For this review, take the finished solid that the model builds, in its own axes (mm). Face numbers are marked on the shaded views. A direction names the side the tool comes from. Round coordinates to 2 decimals unless told otherwise and drop trailing zeros. Order: outer loops, then holes, each group sorted by start corner. A loop starts at its lowest first (then second) coordinate and runs counter-clockwise, first axis right, second up. Notation, with made-up numbers: (-8, 76) -> (21, 76) arc R19 ccw to (21, 109) -> close; hole circle Ø7 at (6, 68). An arc over 180 degrees is marked (long way). Put each result on its own line as item: value. Start each with the question number.
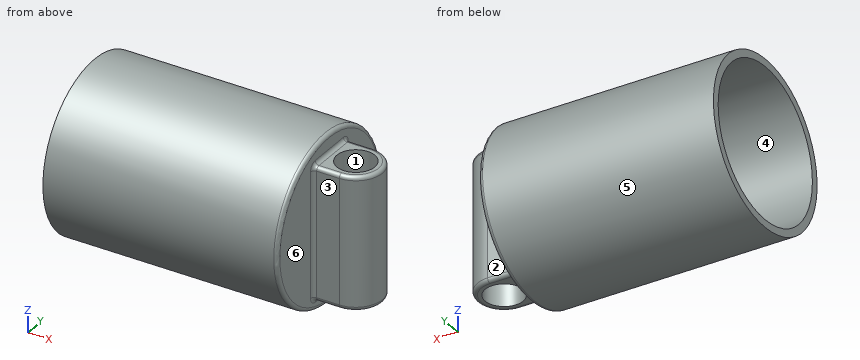
```python
from build123d import *

# Parameters (mm, degrees)
SKETCH3_R           = 5
BOSS_EXTRUDE2_DEPTH = 35
FILLET2_R           = 1
FILLET3_R           = 1


with BuildPart() as part:
    # Sketch1 → Revolve1 (revolve)
    with BuildSketch(Plane.XY, mode=Mode.PRIVATE) as revolve1_sk:
        Polygon((2, 22), (2, 0), (0, 0), (0, 20), (-60, 20), (-60, 22), align=None)
    revolve(revolve1_sk.sketch.rotate(Axis((-25.911369332, 0, 0), (1, 0, 0)), 90), axis=Axis((-25.911369332, 0, 0), (1, 0, 0)))

    # Sketch3 → Boss-Extrude2 (add)
    with BuildSketch(Plane.XY.offset(17)):
        with BuildLine():
            Line((9, 7), (2, 7))
            Line((2, 7), (2, -7))
            Line((2, -7), (9, -7))
            ThreePointArc((9, -7), (16, 0), (9, 7))
        make_face()
        with Locations((9, 0)):
            Circle(SKETCH3_R, mode=Mode.SUBTRACT)
    extrude(amount=-BOSS_EXTRUDE2_DEPTH)

    # Fillet2
    fillet2_edges = [part.edges().sort_by_distance(p)[0] for p in [
        (2, 0, -22),
    ]]
    fillet(fillet2_edges, radius=FILLET2_R)

    # Fillet3
    fillet3_edges = [part.edges().sort_by_distance(p)[0] for p in [
        (16, 0, -18),
        (5.5, -7, -18),
        (2, 0, -18),
        (2, -7, -0.5),
        (5.5, 7, -18),
        (2, 7, -0.5),
        (16, 0, 17),
        (5.5, 7, 17),
        (2, 0, 17),
        (5.5, -7, 17),
    ]]
    fillet(fillet3_edges, radius=FILLET3_R)


solid = part.part
```
Item 1: Consider section C-C, the plane x = 7.5. Write out the cut boundary in (y, z), plus the area to 3 significant figures.
Item 2: Consider section D-D, the plane x = -44. Write out the cut boundary in (y, z).
Item 3: Tool access review of the marked faces 1, 2 and 3: name each direction out of +Z, -Z, +X, -X, +Y, -Y from which nothing blocks a thin tool from reaching the whole face with its end or side.
Item 4: Consider section B-B, the plane z = 0. Write out the cut boundary in (x, y), plus the area to 3 significant figures.
Item 5: For L1, parallel to Y at x = -44.5, z = -0.5; L2, parallel to Y at x = 9, z = 7; L3, parallel to Z at x = -33, y = -18, list the stretches that pass through material, from the lowest coordinate up.
Item 6: Mouldability with a two-part tool opening along Y and no side actions: class the marked faces 4, 5 and 6 as +Y half, -Y half, draft (parallel to the pull), parting line (faces both ways), or undercut.
Item 7: Consider section A-A, the plane y = 0. Write out the cut boundary in (x, z).
Item 8: Insertion check: pin 1 Ø5 at (x, y) = (-42, 3) entering from -Z; pin 2 Ø1 at (x, y) = (-50, -13) entering from -Z; pin 3 Ø21 at (y, z) = (-9, -10.5) entering from +X; pin 4 Ø11.5 at (x, y) = (9, 0) entering from +Z. Each pin has a flat end and moves straight along its axis. Give the tip position at first contact, or say it passes through.
Evaluation:
1. outline: (-7, -17) arc R1 ccw to (-6, -18) -> (-4.77, -18) -> (-4.77, 17) -> (-6, 17) arc R1 ccw to (-7, 16) -> close; (4.77, -18) -> (6, -18) arc R1 ccw to (7, -17) -> (7, 16) arc R1 ccw to (6, 17) -> (4.77, 17) -> close
1. area: 155 mm^2
2. outline: circle Ø44 at (0, 0); hole circle Ø40 at (0, 0)
3. face 1: +Z, -Z
3. face 2: +Z, -Z, +X, +Y
3. face 3: +Z, -Z, +X, -Y
4. outline: (-60, -22) -> (1, -22) arc R1 ccw to (2, -21) -> (2, -8) arc R1 cw to (3, -7) -> (9, -7) arc R7 ccw to (9, 7) -> (3, 7) arc R1 cw to (2, 8) -> (2, 21) arc R1 ccw to (1, 22) -> (-60, 22) -> (-60, 20) -> (0, 20) -> (0, -20) -> (-60, -20) -> close; hole circle Ø10 at (9, 0)
4. area: 424 mm^2
5. L1: y = -21.99 to -19.99, 19.99 to 21.99
5. L2: y = -7 to -5, 5 to 7
5. L3: z = -12.65 to -8.72, 8.72 to 12.65
6. face 4: undercut
6. face 5: parting line
6. face 6: draft
7. outline: (-60, -22) -> (1, -22) arc R1 ccw to (2, -21) -> (2, -19) arc R1 cw to (3, -18) -> (4, -18) -> (4, 17) -> (3, 17) arc R1 cw to (2, 18) -> (2, 21) arc R1 ccw to (1, 22) -> (-60, 22) -> (-60, 20) -> (0, 20) -> (0, -20) -> (-60, -20) -> close; (14, -18) -> (15, -18) arc R1 ccw to (16, -17) -> (16, 16) arc R1 ccw to (15, 17) -> (14, 17) -> close
8. pin 1: stops at z = -21.99
8. pin 2: stops at z = -18.1
8. pin 3: stops at x = 16
8. pin 4: stops at z = 17
